from build123d import *

# Parameters (mm, degrees)
F0_W        = 83.1117276102
F0_H        = 55.7723436505
F1_DEPTH    = 25.4
F2_T        = 2.54
F3_T1_DEPTH = 53.34
F5_D        = 16.66748
F5_DEPTH    = 56.4907174323
F6_W        = 0.9412951767
F6_H        = 22.3557362333
F7_DEPTH    = 25.4


# Not quite as in the source:
# - a fillet or chamfer that OpenCascade refuses, or shapes differently, is made with other operations: its cross-section is extruded or revolved along the edge and cut away or added


with BuildPart() as f1:
    # F0 (on Front) → F1 (new body)
    with BuildSketch(Plane.XZ):
        with Locations((12.3938536271, -8.5663376376)):
            Rectangle(F0_W, F0_H)
    extrude(amount=F1_DEPTH)

    # F2
    f2_openings = [f1.faces().sort_by_distance(p)[0] for p in [
        (12.393854, -25.4, -8.566338),
    ]]
    offset(amount=F2_T, openings=f2_openings, kind=Kind.INTERSECTION)

    # F3: fillet of radius 5.08 on 4 edges, made by hand

    # F3_s2 → F3_t1 (cut)
    with BuildSketch(Plane.XZ.offset(-15.24)):
        with BuildLine():
            ThreePointArc((51.4097174323, 21.8598341876), (55.0018198807, 20.3719366361), (56.4897174323, 16.7798341876))
            Line((56.4897174323, 16.7798341876), (56.4897174323, 21.8598341876))
            Line((56.4897174323, 21.8598341876), (51.4097174323, 21.8598341876))
        make_face()
        with BuildLine():
            ThreePointArc((-26.622010178, 21.8598341876), (-30.2141126264, 20.3719366361), (-31.702010178, 16.7798341876))
            Line((-31.702010178, 16.7798341876), (-31.702010178, 21.8598341876))
            Line((-31.702010178, 21.8598341876), (-26.622010178, 21.8598341876))
        make_face()
        with BuildLine():
            ThreePointArc((-31.702010178, -33.9125094628), (-30.2141126264, -37.5046119113), (-26.622010178, -38.9925094628))
            Line((-26.622010178, -38.9925094628), (-31.702010178, -38.9925094628))
            Line((-31.702010178, -38.9925094628), (-31.702010178, -33.9125094628))
        make_face()
        with BuildLine():
            ThreePointArc((51.4097174323, -38.9925094628), (55.0018198807, -37.5046119113), (56.4897174323, -33.9125094628))
            Line((56.4897174323, -33.9125094628), (56.4897174323, -38.9925094628))
            Line((56.4897174323, -38.9925094628), (51.4097174323, -38.9925094628))
        make_face()
    extrude(amount=F3_T1_DEPTH, mode=Mode.SUBTRACT)

    # F5 (through all, one way)
    with BuildSketch(Plane(origin=(0, 0, 0), x_dir=(0, 1, 0), z_dir=(-1, 0, 0))):
        with Locations((-11.7502789944, -7.3858899996)):
            Circle(F5_D / 2)
    extrude(amount=-F5_DEPTH, mode=Mode.SUBTRACT)

    # F6 (on Front) → F7 (join)
    with BuildSketch(Plane.XZ):
        with Locations((-26.8268827349, -2.7062208392)):
            Rectangle(F6_W, F6_H)
    extrude(amount=F7_DEPTH)


solid = f1.part
Build history of the part. All positions in model axes, mm. A direction names the side the tool comes from. Give positions to 0.01 mm unless a question says otherwise; leave off trailing zeros. Order: outer loops, then holes, each group sorted by start corner. A loop starts at its lowest first (then second) coordinate and runs counter-clockwise, first axis right, second up. Notation, with made-up numbers: M -30.75,1.5 L -12.75,1.5 A18 cw -12.75,8.5 Z; hole C 19,29 d9. An arc over 180 degrees is marked long. Use one line per item in the form item = value.
1) Two-plate mould, pull along X, no slides. Class faces 4 (the face through (12, -11, 21.86)), 5 (the face through (-30.174, -11.234, 20.411)), 6 (the face through (12, -13, -36.453)): released by +X, released by -X, zero draft, split by the parting line, or undercut.
Calculated:
face_4 = zero draft
face_5 = released by -X
face_6 = undercut
2) Probe probe 1 along X at (y, z) = (-13.5, -9); probe 2 along Z at (x, y) = (21, -4.5); probe 3 along X at (y, z) = (-16, -21.5). List the from-to ranges inside material, lowest first.
Calculated:
probe_1 = -31.7 to -29.16, -27.3 to -26.36, 53.95 to 56.49
probe_2 = -38.99 to -36.45, 19.32 to 21.86
probe_3 = -31.7 to -29.16, 53.95 to 56.49
3) Saw through at A-A (y = -15.25). Give the cut face in (x, z).
Calculated:
outline = M -31.7,-33.91 A5.08 ccw -26.62,-38.99 L 51.41,-38.99 A5.08 ccw 56.49,-33.91 L 56.49,-0.18 L 53.95,-0.18 L 53.95,-36.45 L -29.16,-36.45 L -29.16,19.32 L 53.95,19.32 L 53.95,14.95 L 56.49,14.95 L 56.49,16.78 A5.08 ccw 51.41,21.86 L -26.62,21.86 A5.08 ccw -31.7,16.78 Z; M -27.3,-13.88 L -26.36,-13.88 L -26.36,8.47 L -27.3,8.47 Z
4) Saw through at B-B (z = -17). Give the cut face in (x, y).
Calculated:
outline = M -31.7,-25.4 L -29.16,-25.4 L -29.16,0 L 53.95,0 L 53.95,-25.4 L 56.49,-25.4 L 56.49,2.54 L -31.7,2.54 Z
5) Saw through at C-C (x = -18.5). Give the cut face in (y, z), plus the area to 3 significant figures.
Calculated:
outline = M -25.4,-38.99 L 2.54,-38.99 L 2.54,21.86 L -25.4,21.86 L -25.4,19.32 L 0,19.32 L 0,-36.45 L -25.4,-36.45 Z
area = 284 mm2
6) Drop a flat-ended pin along its axis: pin 1 (10 mm diameter, centred on x = 31, z = 2, fed in from -Y). Give the stop position or say it passes through.
Calculated:
pin_1 = 0
7) Saw through at D-D (z = 11). Give the cut face in (x, y), plus the area to 3 significant figures.
Calculated:
outline = M -31.7,-25.4 L -29.16,-25.4 L -29.16,0 L 53.95,0 L 53.95,-4.24 L 56.49,-4.24 L 56.49,2.54 L -31.7,2.54 Z; M 53.95,-25.4 L 56.49,-25.4 L 56.49,-19.26 L 53.95,-19.26 Z
area = 315 mm2
8) Tool access for faces 1 (the face through (55.202, -4.052, 10.578)), 2 (the face through (53.95, -13, -9)), 3 (the face through (-31.702, -11, -9)): list every direction of +Z, -Z, +X, -X, +Y, -Y with a clear straight run to the whole face (end or side of a thin tool).
Calculated:
face_1 = +X
face_2 = -Y
face_3 = +Z, -Z, -X, +Y, -Y
